Part model, mm, in its own coordinate system. A direction names the side the tool comes from. Give positions to 0.01 mm unless a question says otherwise; leave off trailing zeros. Order: outer loops, then holes, each group sorted by start corner. A loop starts at its lowest first (then second) coordinate and runs counter-clockwise, first axis right, second up. Notation, with made-up numbers: (-11, 57.5) -> (19, 57.5) arc R9 ccw to (19, 63.5) -> close; hole circle Ø7 at (38.5, -33.75). An arc over 180 degrees is marked (long way). Write item = value, one per line. Start each with the question number.
(1) Saw through at B-B, the plane y = 6.5. List the corners of the cut face in (x, z).
(2) Saw through at A-A, the plane y = 4.25. List the corners of the cut face in (x, z), then the cut area to 3 significant figures.
(3) Which spindle directions (+Z, -Z, +X, -X, +Y, -Y) get a long thin tool onto all of the face, cutting with end or side? Do faces 1 (the cylindrical face through (2.627, 9.715, -1.552)), 2 (the flat face through (-2.46, 4.44, -9.34)). Say none if no direction does.
(4) Flat gauge pins, fed straight in: pin 1 (5 mm diameter, centred on y = 3.5, z = -5, fed in from -X); pin 2 (1.5 mm diameter, centred on x = -6, y = 5.5, fed in from -Z); pin 3 (3 mm diameter, centred on x = -1, z = -1.5, fed in from +Y); pin 4 (6 mm diameter, centred on y = 2, z = -2.5, fed in from -X). Where does each tip first touch, or does it go through?
(5) Two-plate mould, pull along Z, no slides. Class faces 3 (the cylindrical face through (-2.627, 9.715, 1.552)), 4 (the cylindrical face through (2.387, 9.715, -9.049)), 5 (the cylindrical face through (2.457, 9.715, 9.03)): pulls with the +Z half, pulls with the -Z half, needs draft (parallel to the pull), parting line crosses it, or undercut.
(6) Saw through at C-C, the plane y = 9.25. List the corners of the cut face in (x, z), then the cut area to 3 significant figures.
(7) Probe line 1 along Z through (x, y) = (0, 3.5); line 2 along X through (y, z) = (6.5, 1). List the from-to ranges inside material, lowest first. Write a range as from..to.
from build123d import *

# Parameters (mm, degrees)
SKETCH1_R           = 1.6
BOSS_EXTRUDE1_DEPTH = 10
CUT_EXTRUDE1_DEPTH  = 5
FILLET1_R           = 1


with BuildPart() as part:
    # Sketch1 → Boss-Extrude1 (new body)
    with BuildSketch(Plane(origin=(0, 0, 0), x_dir=(1, 0, 0), z_dir=(0, 1, 0))):
        Polygon((-10, 0), (-8.660254038, -5), (-5, -8.660254038), (0, -10), (5, -8.660254038), (8.660254038, -5), (10, 0), (8.660254038, 5), (5, 8.660254038), (0, 10), (-5, 8.660254038), (-8.660254038, 5), align=None)
        with Locations(Location((0, 0, 0), (0, 0, 270))):
            Circle(SKETCH1_R, mode=Mode.SUBTRACT)
    extrude(amount=BOSS_EXTRUDE1_DEPTH)

    # Sketch2 → Cut-Extrude1 (cut)
    with BuildSketch(Plane(origin=(0, 10, 0), x_dir=(1, 0, 0), z_dir=(0, 1, 0))):
        Polygon((3.175426481, 0), (1.58771324, 2.75), (-1.58771324, 2.75), (-3.175426481, 0), (-1.58771324, -2.75), (1.58771324, -2.75), align=None)
    extrude(amount=-CUT_EXTRUDE1_DEPTH, mode=Mode.SUBTRACT)

    # Fillet1
    fillet1_edges = [part.edges().sort_by_distance(p)[0] for p in [
        (9.330127019, 10, -2.5),
        (6.830127019, 10, -6.830127019),
        (2.5, 10, -9.330127019),
        (-2.5, 10, -9.330127019),
        (-6.830127019, 10, -6.830127019),
        (-9.330127019, 10, -2.5),
        (-9.330127019, 10, 2.5),
        (-6.830127019, 10, 6.830127019),
        (-2.5, 10, 9.330127019),
        (2.38156986, 10, 1.375),
        (2.38156986, 10, -1.375),
        (0, 10, -2.75),
        (-2.38156986, 10, -1.375),
        (-2.38156986, 10, 1.375),
        (0, 10, 2.75),
        (2.5, 10, 9.330127019),
        (6.830127019, 10, 6.830127019),
        (9.330127019, 10, 2.5),
    ]]
    fillet(fillet1_edges, radius=FILLET1_R)


solid = part.part
Results list:
q1.outline = (-10, 0) -> (-8.66, -5) -> (-5, -8.66) -> (0, -10) -> (5, -8.66) -> (8.66, -5) -> (10, 0) -> (8.66, 5) -> (5, 8.66) -> (0, 10) -> (-5, 8.66) -> (-8.66, 5) -> close; hole (-3.18, 0) -> (-1.59, -2.75) -> (1.59, -2.75) -> (3.18, 0) -> (1.59, 2.75) -> (-1.59, 2.75) -> close
q2.outline = (-10, 0) -> (-8.66, -5) -> (-5, -8.66) -> (0, -10) -> (5, -8.66) -> (8.66, -5) -> (10, 0) -> (8.66, 5) -> (5, 8.66) -> (0, 10) -> (-5, 8.66) -> (-8.66, 5) -> close; hole circle Ø3.2 at (0, 0)
q2.area = 292 mm^2
q3.face_1 = +Y
q3.face_2 = -Z, -X, +Y, -Y
q4.pin_1 = -9.33
q4.pin_2 = -8.41
q4.pin_3 = 9.77
q4.pin_4 = -10
q5.face_3 = undercut
q5.face_4 = pulls with the -Z half
q5.face_5 = pulls with the +Z half
q6.outline = (-9.97, 0) -> (-8.63, -4.98) -> (-4.98, -8.63) -> (0, -9.97) -> (4.98, -8.63) -> (8.63, -4.98) -> (9.97, 0) -> (8.63, 4.98) -> (4.98, 8.63) -> (0, 9.97) -> (-4.98, 8.63) -> (-8.63, 4.98) -> close; hole (-3.21, 0) -> (-1.61, -2.78) -> (1.61, -2.78) -> (3.21, 0) -> (1.61, 2.78) -> (-1.61, 2.78) -> close
q6.area = 271 mm^2
q7.line_1 = -10..-1.6, 1.6..10
q7.line_2 = -9.73..-2.6, 2.6..9.73
